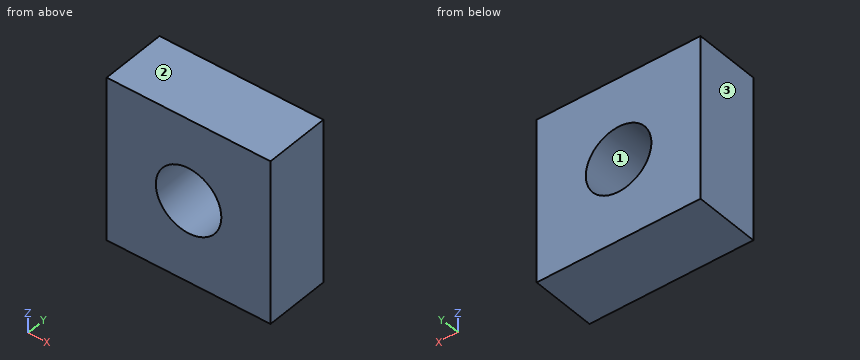
Autodesk Inventor part; units mm, degrees
ref_plane "YZ Plane" through (0, 0, 0) normal (1, 0, 0) x (0, 1, 0)
ref_plane "XZ Plane" through (0, 0, 0) normal (0, 1, 0) x (-1, 0, 0)
ref_plane "XY Plane" through (0, 0, 0) normal (0, 0, 1) x (1, 0, 0)
sketch "Sketch6" plane through (0, 0, 0) normal (0, 1, 0) x (-1, 0, 0)
  line L0 (-3.75, -3.75) -> (3.75, -3.75)
  line L1 (3.75, -3.75) -> (3.75, 3.75)
  line L2 (3.75, 3.75) -> (-3.75, 3.75)
  line L3 (-3.75, 3.75) -> (-3.75, -3.75)
  line L4 (-3.75, -3.75) -> (3.75, 3.75) construction
  line L5 (3.75, -3.75) -> (-3.75, 3.75) construction
  point P0 (0, 0)
  dimension "d4" = 7.5
  dimension "d5" = 7.5
extrude "Extrusion2" add sketch "Sketch6" along normal blind 10
sketch "Sketch7" plane through (3.75, 0, 3.75) normal (1, 0, 0) x (0, 0, -1)
  line L0 (7.5, 0) -> (0, 0)
  line L1 (0, 0) -> (7.5, 0)
  line L2 (0, 0) -> (0, 7)
  line L3 (0, 7) -> (7.5, 7)
  line L4 (7.5, 7) -> (7.5, 0)
  line L5 (7.5, 0) -> (0, 0)
  line L6 (0, 0) -> (0, 10)
  line L7 (7.5, 0) -> (7.5, 10)
  point P0 (3.75, 0)
  dimension "d9" = 7
  dimension "d19" = 0
  dimension "d20" = 0
extrude "Extrusion3" cut sketch "Sketch7" against normal blind 9.05
sketch "Sketch8" plane through (0, 10, 0) normal (0, 1, 0) x (1, 0, 0)
  circle A0 centre (0, 0) radius 1.5
  dimension "d13" = 3
extrude "Extrusion4" cut sketch "Sketch8" against normal blind 5.2375
properties part number "Holder"
Work out the finished part from the listing and answer in its coordinate system (mm). Face numbers are marked on the shaded views. Round coordinates to 2 decimals unless told otherwise and drop trailing zeros. Loops run counter-clockwise (first coordinate to the right, second up) from the corner with the lowest first, then second, coordinate; pieces in that order, holes last.
(1) The mould has two halves that part along Z. Classify the marked faces 1, 2 and 3: pulls with the +Z half, pulls with the -Z half, needs draft (parallel to the pull), parting line crosses it, or undercut.
Computed values:
face 1: undercut
face 2: pulls with the +Z half
face 3: needs draft
(2) The part is cut by section A-A, the plane z = 0. Give the vertices of the cut face in (x, y), and give its area (3 significant figures).
Computed values:
outline: (-3.75, 7) - (-1.5, 7) - (-1.5, 10) - (-3.75, 10) - close; (1.5, 7) - (3.75, 7) - (3.75, 10) - (1.5, 10) - close
area: 13.5 mm2
(3) The part is cut by section C-C, the plane y = 9.25. Give the vertices of the cut face in (x, z), and give its area (3 significant figures).
Computed values:
outline: (-3.75, -3.75) - (3.75, -3.75) - (3.75, 3.75) - (-3.75, 3.75) - close; hole circle Ø3 at (0, 0)
area: 49.2 mm2
(4) The part is cut by section B-B, the plane x = 0. Give the vertices of the cut face in (y, z), and give its area (3 significant figures).
Computed values:
outline: (7, -3.75) - (10, -3.75) - (10, -1.5) - (7, -1.5) - close; (7, 1.5) - (10, 1.5) - (10, 3.75) - (7, 3.75) - close
area: 13.5 mm2
(5) Find the intervals of material crossed by L1, parallel to X at y = 9, z = 0; L2, parallel to X at y = 8.95, z = -0.5, in increasing order.
Computed values:
L1: x = -3.75 to -1.5, 1.5 to 3.75
L2: x = -3.75 to -1.41, 1.41 to 3.75
(6) This flat-tipped pin is pushed along its axis until it touches: P1, Ø3.5, axis at x = 0, z = 0, coming from the +Y side. Where does it stop, or does it pass through?
Computed values:
P1: stops at y = 10
